Design review of the part built by this model. Coordinates are the model's own, in mm. Coordinates: 2 decimals unless noted, no trailing zeros. Order: outer loops, then holes, each group sorted by start corner. A loop starts at its lowest first (then second) coordinate and runs counter-clockwise, first axis right, second up. Notation, with made-up numbers: M 78,85.5 L 103,85.5 A13 ccw 103,101.5 Z; hole C 22.25,89.5 d3. An arc over 180 degrees is marked long. Use CSV: the item, a comma, the result in double quotes.
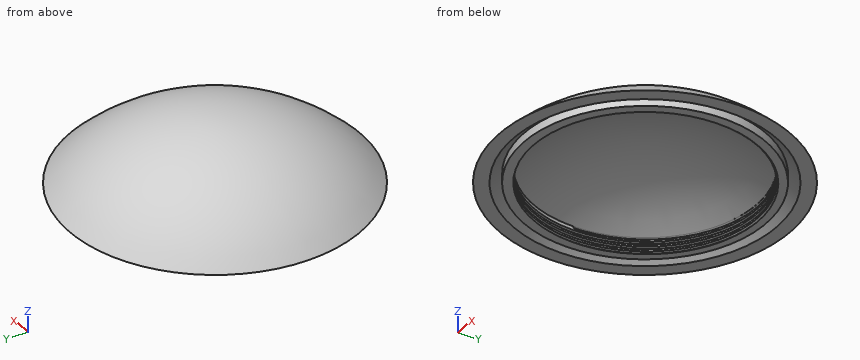
```python
from build123d import *

# Parameters (mm, degrees)
SKETCH2_R                       = 50.9
SKETCH2_R_2                     = 46.9
BOSS_EXTRUDE1_DEPTH             = 5
BOSS_EXTRUDE1_DIRECTION_2_REACH = 90.882
THREAD1_PITCH                   = 2


with BuildPart() as part:
    # Sketch1 → Revolve1 (revolve)
    with BuildSketch(Plane(origin=(0, 0, 0), x_dir=(1, 0, 0), z_dir=(0, 1, 0))):
        with BuildLine():
            ThreePointArc((-61.23724357, -62.5), (-33.071891388, -81.00925873), (0, -87.5))
            Line((0, -87.5), (0, -83.5))
            ThreePointArc((0, -83.5), (-29.609964539, -78.073683146), (-55.3714728, -62.5))
            Line((-55.3714728, -62.5), (-61.23724357, -62.5))
        make_face()
    revolve(axis=Axis((0, 0, 87.5), (0, 0, -1)))

    # Sketch2 → Boss-Extrude1 (add)
    with BuildSketch(Plane(origin=(0, 0, 67.5), x_dir=(-1, 0, 0), z_dir=(0, 0, -1))):
        Circle(SKETCH2_R)
        Circle(SKETCH2_R_2, mode=Mode.SUBTRACT)
    extrude(amount=BOSS_EXTRUDE1_DEPTH)

    # Sketch2 → Boss-Extrude1 direction 2 (add, up to next)
    with BuildSketch(Plane(origin=(0, 0, 67.5), x_dir=(-1, 0, 0), z_dir=(0, 0, -1)), mode=Mode.PRIVATE) as boss_extrude1_direction_2_sk1:
        Circle(SKETCH2_R)
        Circle(SKETCH2_R_2, mode=Mode.SUBTRACT)
    boss_extrude1_direction_2_tool1 = extrude(boss_extrude1_direction_2_sk1.sketch, amount=-BOSS_EXTRUDE1_DIRECTION_2_REACH, mode=Mode.PRIVATE) - part.part
    add(boss_extrude1_direction_2_tool1.solids().sort_by_distance((49.460331, 0, 67.5))[0])

    # Thread1: arcs per turn and ends read off the stored shape
    # Thread1: the profile of Thread Profile1 profile screwed along a right-hand helix through 3.5 turns, 10 arcs to a turn; built about Z, then put on its axis
    thread1_z = Axis((0, 0, 0), (0, 0, 1))
    thread1_corners = [(-46.8997, 0, -7.000173205), (-47.711898812, 0, -6.531250002), (-47.711898812, 0, -6.343750002), (-46.8997, 0, -5.874826799)]
    with BuildLine(mode=Mode.PRIVATE) as thread1_profile:
        Line(thread1_corners[0], thread1_corners[1])
        Line(thread1_corners[1], thread1_corners[2])
        Line(thread1_corners[2], thread1_corners[3])
        Line(thread1_corners[3], thread1_corners[0])
    thread1_cap = Face(thread1_profile.wire())
    thread1_turn_angles = [0, 18, 36, 54, 72, 90, 108, 126, 144, 162, 180, 198, 216, 234, 252, 270, 288, 306, 324, 342, 360]
    thread1_turn_weights = [1, 0.9510565162951535, 1, 0.9510565162951535, 1, 0.9510565162951535, 1, 0.9510565162951535, 1, 0.9510565162951535, 1, 0.9510565162951535, 1, 0.9510565162951535, 1, 0.9510565162951535, 1, 0.9510565162951535, 1, 0.9510565162951535, 1]
    thread1_turn_rails = [Edge.make_bspline([Vector(p[0], p[1], 0).rotate(thread1_z, thread1_turn_angles[k]) / thread1_turn_weights[k] + Vector(0, 0, p[2] + THREAD1_PITCH * thread1_turn_angles[k] / 360) for k in range(21)], [0, 0, 0, 1, 1, 2, 2, 3, 3, 4, 4, 5, 5, 6, 6, 7, 7, 8, 8, 9, 9, 10, 10, 10], 2, thread1_turn_weights) for p in thread1_corners]
    thread1_turn_sides = [Face.make_surface_from_curves(thread1_turn_rails[p[0]], thread1_turn_rails[p[1]]) for p in [(0, 1), (1, 2), (2, 3), (3, 0)]]
    thread1_last_angles = [1080, 1098, 1116, 1134, 1152, 1170, 1188, 1206, 1224, 1242, 1260]
    thread1_last_weights = [1, 0.9510565162951535, 1, 0.9510565162951535, 1, 0.9510565162951535, 1, 0.9510565162951535, 1, 0.9510565162951535, 1]
    thread1_last_rails = [Edge.make_bspline([Vector(p[0], p[1], 0).rotate(thread1_z, thread1_last_angles[k]) / thread1_last_weights[k] + Vector(0, 0, p[2] + THREAD1_PITCH * thread1_last_angles[k] / 360) for k in range(11)], [0, 0, 0, 1, 1, 2, 2, 3, 3, 4, 4, 5, 5, 5], 2, thread1_last_weights) for p in thread1_corners]
    thread1_last_sides = [Face.make_surface_from_curves(thread1_last_rails[p[0]], thread1_last_rails[p[1]]) for p in [(0, 1), (1, 2), (2, 3), (3, 0)]]
    thread1 = Plane(origin=(0, 0, 62.5), x_dir=(1, 0, 0), z_dir=(0, 0, -1)) * Solid(Shell([*[p.moved(Location((0, 0, THREAD1_PITCH * i))) for i in range(3) for p in thread1_turn_sides], *thread1_last_sides, thread1_cap, thread1_cap.rotate(thread1_z, 1260).moved(Location((0, 0, THREAD1_PITCH * 1260 / 360)))]))
    add(thread1, mode=Mode.SUBTRACT)


solid = part.part
```
(1) Add section B-B on z = 76.25. State the section outline as (x, y) points.
The answers:
outline,"C 0,0 d85.84; hole C 0,0 d68.06"
(2) Add section A-A on x = -53. State the section outline as (y, z) points, and give its area (3 significant figures).
The answers:
outline,"M -30.68,62.5 L -16.03,62.5 A64.52 cw 16.03,62.5 L 30.68,62.5 A69.62 ccw Z"
area,"251 mm2"
(3) Clearance check with flat-ended pins moving along their axes: P1, Ø3, axis at x = 3, y = -47, coming from the +Z side; P2, Ø4, axis at y = 21.5, z = 79, coming from the -X side; P3, Ø5, axis at x = 30.5, y = 2, coming from the +Z side. State where each tip first meets the part, or that it passes through.
The answers:
P1,"stops at z = 74.68"
P2,"stops at x = -35.73"
P3,"stops at z = 82.88"
(4) Wall thickness on probe 1 along X at (y, z) = (0, 65.15); probe 2 along X at (y, z) = (0, 64.5); probe 3 along Y at (x, z) = (0, 65.7): over which ranges is each line inside the solid? List them lowest first.
The answers:
probe 1,"x = -58.41 to -52.23, -50.9 to -47.51, 46.9 to 50.9, 52.23 to 58.41"
probe 2,"x = -59.13 to -53.03, -50.9 to -47.12, 46.9 to 50.9, 53.03 to 59.13"
probe 3,"y = -57.79 to -51.53, -50.9 to -47.42, 46.9 to 50.9, 51.53 to 57.79"
